Check sheet for the modelled part. Datum: model origin and axes. Units: mm. Face numbers are marked on the shaded views. A direction names the side the tool comes from. Give positions to 0.01 mm unless a question says otherwise; leave off trailing zeros. Write each loop counter-clockwise with the first axis right and the second up, starting at its lowest first coordinate (ties: lowest second). Pieces come first, ordered by that corner, then holes. Notation, with made-up numbers: (51, 14) -> (76, 14) arc R25 ccw to (76, 51) -> close; hole circle Ø9 at (-11, 83). An arc over 180 degrees is marked (long way). Use a Markdown table: item, result. Add a question column.
1. Scan lines: probe 1 along Y at (x, z) = (-5, 0.95); probe 2 along X at (y, z) = (6, 0.3); probe 3 along Y at (x, z) = (0, 2.45). Record each from-to range of solid material in increasing order. Write a range as [from, to].
2. Release check for a two-part mould opening along Y. For the marked faces 1, 2 and 3 record: released by +Y, released by -Y, zero draft, split by the parting line, or undercut.
3. Set-up check for the marked faces 4 and 5: record each of +Z, -Z, +X, -X, +Y, -Y from which the full face is reachable in a straight line by a thin tool's end or side.
4. Cross-section at B-B (y = -5). Enter the section's corners in (x, z), then the cut area to 3 significant figures.
5. Gauge pin test, flat ends, axial feed: P1, Ø1.5, axis at x = -5, y = 3, coming from the -Z side; P2, Ø3, axis at x = -5, y = 5, coming from the +Z side; P3, Ø1.5, axis at x = 2.5, z = 0.5, coming from the +Y side. Record the tip position at first contact, or that the pin passes through.
6. Cross-section at C-C (z = 0.3). Count the separate pieces of the cut face and the enclosed holes in it, then the cut area to 3 significant figures.
7. Cross-section at D-D (x = -6). Enter the section's corners in (y, z), then the cut area to 3 significant figures.
8. Cross-section at A-A (x = 0). Enter the section's corners in (y, z), then the cut area to 3 significant figures.
Autodesk Inventor part; units mm, degrees
ref_plane "YZ Plane" through (0, 0, 0) normal (1, 0, 0) x (0, 1, 0)
ref_plane "XZ Plane" through (0, 0, 0) normal (0, 1, 0) x (-1, 0, 0)
ref_plane "XY Plane" through (0, 0, 0) normal (0, 0, 1) x (1, 0, 0)
sketch "スケッチ1" plane through (0, 0, 0) normal (0, 0, 1) x (1, 0, 0)
  circle A0 centre (0, 0) radius 10
  dimension "d0" = 20
extrude "押し出し1" add sketch "スケッチ1" along normal blind 2.2
sketch "スケッチ2" plane through (0, 0, 2.2) normal (0, 0, 1) x (1, 0, 0)
  circle A0 centre (0, 0) radius 4.5
  dimension "d3" = 9
extrude "押し出し2" add sketch "スケッチ2" along normal blind 1.3
sketch "スケッチ3" plane through (0, 0, 0) normal (0, 0, -1) x (-1, 0, 0)
  circle A0 centre (0, 0) radius 10
  line L0 (0, 10) -> (0, -10)
  line L1 (-10, 0) -> (10, 0)
  point P0 (-5, 5)
  point P1 (5, 5)
  point P2 (5, -5)
  point P3 (-5, -5)
  dimension "d6" = 10
  dimension "d7" = 10
hole "穴1" at (5, 5, 0) at (-5, 5, 0) at (-5, -5, 0) at (5, -5, 0) direction (0, 0, 1) diameter 2.459 end through all
sketch "スケッチ4" plane through (0, 0, 3.5) normal (0, 0, -1) x (-1, 0, 0)
  point P0 (0, 0)
  point P1 (0, 0)
hole "穴2" at (0, 0, 3.5) direction (0, 0, -1) diameter 6 end through all
sketch "スケッチ5" plane through (0, 0, 0) normal (0, 0, -1) x (-1, 0, 0)
  point P0 (-2.7296, -6.523)
  point P1 (2.7296, 6.523)
  point P2 (-6.523, 2.7296)
  point P3 (6.523, -2.7296)
hole "穴3" at (2.7296, -6.523, 0) at (-2.7296, 6.523, 0) at (6.523, 2.7296, 0) at (-6.523, -2.7296, 0) direction (0, 0, 1) diameter 2.459 depth 7 tip angle 120
properties part number "サーボモータ25kgcmサーボホーン1" material "アルミニウム 6061"
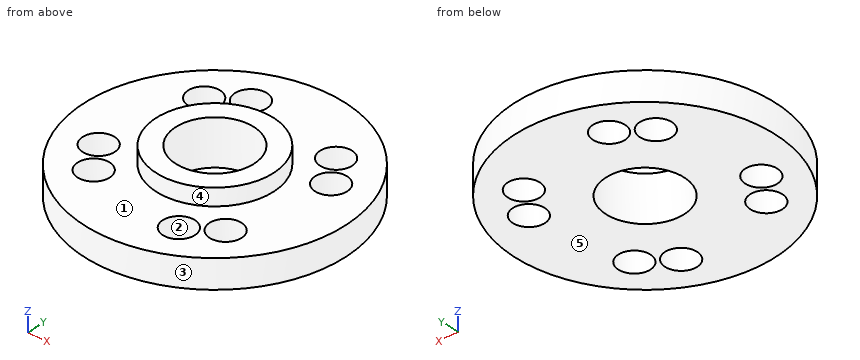
Worked answers:
| question | item | result |
|---|---|---|
| 1 | probe 1 | y = [-8.66, -6.23], [-3.77, 3.77], [6.23, 8.66] |
| 1 | probe 2 | x = [-8, -5.72], [-4.28, -3.84], [-1.62, 4.28], [5.72, 8] |
| 1 | probe 3 | y = [-4.5, -3], [3, 4.5] |
| 2 | face 1 | zero draft |
| 2 | face 2 | undercut |
| 2 | face 3 | split by the parting line |
| 3 | face 4 | +Z |
| 3 | face 5 | -Z, +X, -X, +Y, -Y |
| 4 | outline | (-8.66, 0) -> (-6.23, 0) -> (-6.23, 2.2) -> (-8.66, 2.2) -> close; (-3.77, 0) -> (3.77, 0) -> (3.77, 2.2) -> (-3.77, 2.2) -> close; (6.23, 0) -> (8.66, 0) -> (8.66, 2.2) -> (6.23, 2.2) -> close |
| 4 | area | 27.3 mm² |
| 5 | P1 | stops at z = 0 |
| 5 | P2 | stops at z = 2.2 |
| 5 | P3 | stops at y = 9.85 |
| 6 | separate pieces | 1 |
| 6 | enclosed holes | 9 |
| 6 | area | 248 mm² |
| 7 | outline | (-8, 0) -> (-5.72, 0) -> (-5.72, 2.2) -> (-8, 2.2) -> close; (-4.28, 0) -> (-3.84, 0) -> (-3.84, 2.2) -> (-4.28, 2.2) -> close; (-1.62, 0) -> (4.28, 0) -> (4.28, 2.2) -> (-1.62, 2.2) -> close; (5.72, 0) -> (8, 0) -> (8, 2.2) -> (5.72, 2.2) -> close |
| 7 | area | 24.0 mm² |
| 8 | outline | (-10, 0) -> (-3, 0) -> (-3, 3.5) -> (-4.5, 3.5) -> (-4.5, 2.2) -> (-10, 2.2) -> close; (3, 0) -> (10, 0) -> (10, 2.2) -> (4.5, 2.2) -> (4.5, 3.5) -> (3, 3.5) -> close |
| 8 | area | 34.7 mm² |
